The listing builds one solid part. Answer for the finished solid, in the listing's coordinates (mm). Face numbers are marked on the shaded views. A direction names the side the tool comes from. Round coordinates to 2 decimals unless told otherwise and drop trailing zeros. Loops run counter-clockwise (first coordinate to the right, second up) from the corner with the lowest first, then second, coordinate; pieces in that order, holes last. Notation, with made-up numbers: (9.5, 71) -> (30.5, 71) arc R29 cw to (30.5, 104) -> close; hole circle Ø1 at (10, -13). An arc over 180 degrees is marked (long way). Use a Markdown table: item, result. Add a question column.
Q1. Section B-B on y = 132 is taken. Give the vertices of the cut face in (x, z).
Q2. Section D-D on x = -114.5 is taken. Give the vertices of the cut face in (y, z).
Q3. Section A-A on x = 0 is taken. Give the vertices of the cut face in (y, z).
Q4. Section C-C on z = 53 is taken. Give the vertices of the cut face in (x, y).
Q5. Given pin 1 Ø10 at (x, z) = (-31.5, -36.5) entering from +Y; pin 2 Ø10 at (x, z) = (-119.5, 24.5) entering from +Y; pin 3 Ø1 at (x, y) = (12, 13) entering from -Z, each flat-ended and moving along its own axis, determine where each tip first touches the part or whether it passes through.
Q6. For a pull along Y with two mould halves and no side action, classify the marked faces 4, 5, 6 and 7 as released by +Y, released by -Y, zero draft, split by the parting line, or undercut.
Q7. Which of the six approach directions +Z, -Z, +X, -X, +Y, -Y give full straight-line access (tool end or side, diameter ignored) to the marked faces 1, 2 and 3?
Q8. Consider line 1 (Y direction, x = -4, z = -1.5); line 2 (X direction, y = 3, z = -44); line 3 (X direction, y = 58.5, z = 8). Determine where each line is inside the solid, lowest interval first.
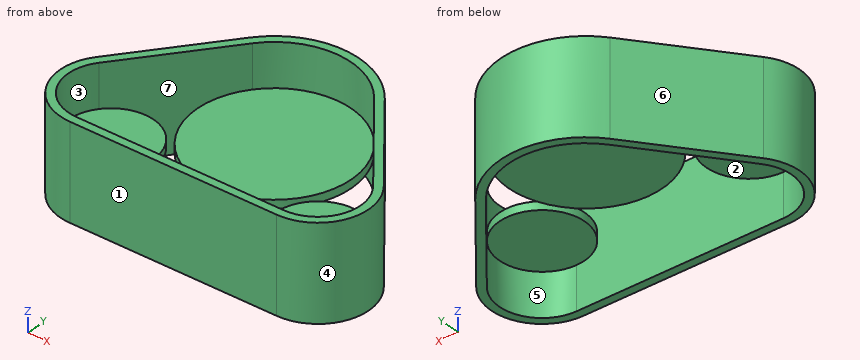
from build123d import *

# Parameters (mm, degrees)
SCHIZZO1_R                     = 52
ESTRUSIONE_ESTRUSIONE1_DEPTH   = 10
ESTRUSIONE_ESTRUSIONE1_2_DEPTH = 10
SCHIZZO1_R_2                   = 94
ESTRUSIONE_ESTRUSIONE1_3_DEPTH = 10
ESTRUSIONE_SOTTILE1_DEPTH      = 52.5
ESTRUSIONE_SOTTILE1_DEPTH_BACK = 62.5


with BuildPart() as part:
    # Schizzo1 → Estrusione-Estrusione1 (new body)
    with BuildSketch(Plane.XY):
        with Locations((-125, 0)):
            Circle(SCHIZZO1_R)
    extrude(amount=ESTRUSIONE_ESTRUSIONE1_DEPTH)



with BuildPart() as body_2:
    # Schizzo1 → Estrusione-Estrusione1 2 (new body)
    with BuildSketch(Plane.XY):
        with Locations((125, 0)):
            Circle(SCHIZZO1_R)
    extrude(amount=ESTRUSIONE_ESTRUSIONE1_2_DEPTH)


with BuildPart() as body_3:
    # Schizzo1 → Estrusione-Estrusione1 3 (new body)
    with BuildSketch(Plane.XY):
        with Locations((0, 90)):
            Circle(SCHIZZO1_R_2)
    extrude(amount=ESTRUSIONE_ESTRUSIONE1_3_DEPTH)


with BuildPart() as part_1:
    add(part.part)

    add(body_2.part)  # Estrusione-Sottile1 merges body 2

    add(body_3.part)  # Estrusione-Sottile1 merges body 3
    # Schizzo2 → Estrusione-Sottile1 (add, two sides: drawn at the far end of the back side and taken through both)
    with BuildSketch(Plane.XY.offset(10).offset(-ESTRUSIONE_SOTTILE1_DEPTH_BACK)):
        with BuildLine():
            Line((81.478662228, 154.631475316), (173.573817867, 38.530302592))
            ThreePointArc((173.573817867, 38.530302592), (180.825078418, -26.973331638), (125, -62))
            Line((125, -62), (-125, -62))
            ThreePointArc((-125, -62), (-180.825078418, -26.973331638), (-173.573817867, 38.530302592))
            Line((-173.573817867, 38.530302592), (-81.478662228, 154.631475316))
            ThreePointArc((-81.478662228, 154.631475316), (0, 194), (81.478662228, 154.631475316))
        make_face()
        with BuildLine():
            Line((73.644175475, 148.416910382), (165.739331114, 32.315737658))
            ThreePointArc((165.739331114, 32.315737658), (171.821033512, -22.622794277), (125, -52))
            Line((125, -52), (-125, -52))
            ThreePointArc((-125, -52), (-171.821033512, -22.622794277), (-165.739331114, 32.315737658))
            Line((-165.739331114, 32.315737658), (-73.644175475, 148.416910382))
            ThreePointArc((-73.644175475, 148.416910382), (0, 184), (73.644175475, 148.416910382))
        make_face(mode=Mode.SUBTRACT)
    extrude(amount=ESTRUSIONE_SOTTILE1_DEPTH + ESTRUSIONE_SOTTILE1_DEPTH_BACK)


solid = part_1.part
Checked values:
| question | item | result |
|---|---|---|
| 1 | outline | (-99.43, -52.5) -> (-86.67, -52.5) -> (-86.67, 62.5) -> (-99.43, 62.5) -> close; (-84.1, 0) -> (84.1, 0) -> (84.1, 10) -> (-84.1, 10) -> close; (86.67, -52.5) -> (99.43, -52.5) -> (99.43, 62.5) -> (86.67, 62.5) -> close |
| 2 | outline | (-62, -52.5) -> (-52, -52.5) -> (-52, 62.5) -> (-62, 62.5) -> close; (-50.93, 0) -> (50.93, 0) -> (50.93, 10) -> (-50.93, 10) -> close; (96.91, -52.5) -> (113, -52.5) -> (113, 62.5) -> (96.91, 62.5) -> close |
| 3 | outline | (-62, -52.5) -> (-52, -52.5) -> (-52, 62.5) -> (-62, 62.5) -> close; (-4, 0) -> (184, 0) -> (184, -52.5) -> (194, -52.5) -> (194, 62.5) -> (184, 62.5) -> (184, 10) -> (-4, 10) -> close |
| 4 | outline | (-173.57, 38.53) arc R62 ccw to (-125, -62) -> (125, -62) arc R62 ccw to (173.57, 38.53) -> (81.48, 154.63) arc R104 ccw to (-81.48, 154.63) -> close; hole (-165.74, 32.32) arc R52 ccw to (-125, -52) -> (125, -52) arc R52 ccw to (165.74, 32.32) -> (73.64, 148.42) arc R94 ccw to (-73.64, 148.42) -> close |
| 5 | pin 1 | stops at y = 190.57 |
| 5 | pin 2 | stops at y = 113 |
| 5 | pin 3 | stops at z = 0 |
| 6 | face 4 | split by the parting line |
| 6 | face 5 | undercut |
| 6 | face 6 | released by +Y |
| 6 | face 7 | undercut |
| 7 | face 1 | +Z, -Z, +X, -X, -Y |
| 7 | face 2 | -Z |
| 7 | face 3 | +Z |
| 8 | line 1 | y = -62 to -52, 183.91 to 193.92 |
| 8 | line 2 | x = -186.93 to -176.91, 176.91 to 186.93 |
| 8 | line 3 | x = -157.73 to -144.97, -88.56 to 88.56, 144.97 to 157.73 |
